Work out the finished part from the listing and answer in its coordinate system (mm). Give positions to 0.01 mm unless a question says otherwise; leave off trailing zeros. Write each loop counter-clockwise with the first axis right and the second up, starting at its lowest first coordinate (ties: lowest second). Pieces come first, ordered by that corner, then holes. Notation, with made-up numbers: (15.5, 60) -> (38.5, 60) arc R19 cw to (38.5, 68) -> close; hole circle Ø3 at (-21.75, 88). An arc over 180 degrees is marked (long way). Use a Markdown table: item, result. Add a question column.
Q1. Section D-D, the plane z = 19.5 is taken. Give the vertices of the cut face in (x, y), plus the area to 3 significant figures.
Q2. Each of these flat-tipped pins is pushed along its axis until it touches: pin 1 Ø5.5 at (x, y) = (17.5, -51) entering from -Z; pin 2 Ø5.5 at (y, z) = (1, -116) entering from -X; pin 3 Ø5.5 at (y, z) = (-50.5, -151.5) entering from +X; pin 4 Ø10 at (x, z) = (-24.5, -42.5) entering from +Y. Where does it stop, or does it pass through?
Q3. Section A-A, the plane y = -44 is taken. Give the vertices of the cut face in (x, z).
Q4. Section C-C, the plane x = 19 is taken. State how many separate pieces and enclosed holes the cut face has, plus the area to 3 significant figures.
Q5. Consider line 1 (Z direction, x = 0, y = 1); line 2 (Z direction, x = 0, y = -35.25); line 3 (X direction, y = -17, z = 0). Determine where each line is inside the solid, lowest interval first.
Q6. Section B-B, the plane z = -150 is taken. Give the vertices of the cut face in (x, y).
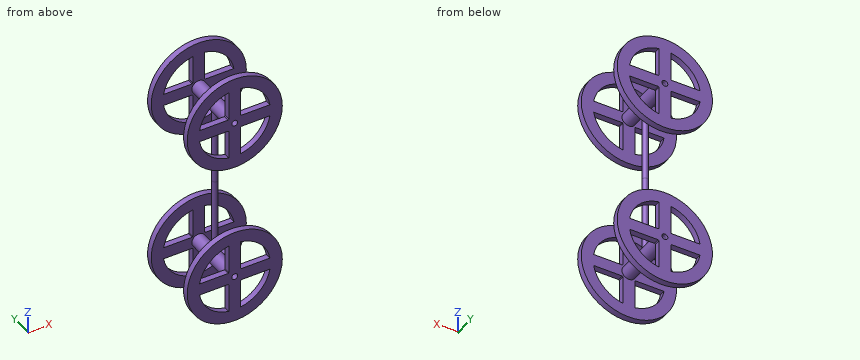
from build123d import *

# Parameters (mm, degrees)
F0_R     = 40
F1_DEPTH = 2.5
F2_R     = 5.8113961387
F2_R_2   = 3.4738590418
F3_DEPTH = 25


with BuildPart() as f1:
    # F0 (on Front) → F1 (new body, symmetric)
    with BuildSketch(Plane.XZ):
        Circle(F0_R)
        with BuildLine():
            Line((-29.5803989155, -5), (-5.5901699437, -5))
            ThreePointArc((-5.5901699437, -5), (-5.3033008589, -5.3033008589), (-5, -5.5901699437))
            Line((-5, -5.5901699437), (-5, -29.5803989155))
            ThreePointArc((-5, -29.5803989155), (-21.2132034356, -21.2132034356), (-29.5803989155, -5))
        make_face(mode=Mode.SUBTRACT)
        with BuildLine():
            Line((5, -29.5803989155), (5, -5.5901699437))
            ThreePointArc((5, -5.5901699437), (5.3033008589, -5.3033008589), (5.5901699437, -5))
            Line((5.5901699437, -5), (29.5803989155, -5))
            ThreePointArc((29.5803989155, -5), (21.2132034356, -21.2132034356), (5, -29.5803989155))
        make_face(mode=Mode.SUBTRACT)
        with BuildLine():
            Line((-5, 29.5803989155), (-5, 5.5901699437))
            ThreePointArc((-5, 5.5901699437), (-5.3033008589, 5.3033008589), (-5.5901699437, 5))
            Line((-5.5901699437, 5), (-29.5803989155, 5))
            ThreePointArc((-29.5803989155, 5), (-21.2132034356, 21.2132034356), (-5, 29.5803989155))
        make_face(mode=Mode.SUBTRACT)
        with BuildLine():
            ThreePointArc((0, -2.5), (-1.767766953, 1.767766953), (2.5, 0))
            ThreePointArc((2.5, 0), (1.767766953, -1.767766953), (0, -2.5))
        make_face(mode=Mode.SUBTRACT)
        with BuildLine():
            ThreePointArc((5, 29.5803989155), (21.2132034356, 21.2132034356), (29.5803989155, 5))
            Line((29.5803989155, 5), (5.5901699437, 5))
            ThreePointArc((5.5901699437, 5), (5.3033008589, 5.3033008589), (5, 5.5901699437))
            Line((5, 5.5901699437), (5, 29.5803989155))
        make_face(mode=Mode.SUBTRACT)
    extrude(amount=F1_DEPTH, both=True)

    # F2 (on Front) → F3 (join)
    with BuildSketch(Plane.XZ):
        Circle(F2_R)
        Circle(F2_R_2, mode=Mode.SUBTRACT)
    extrude(amount=F3_DEPTH)

    # F4: F1 across face


with BuildPart() as f1_1:
    add(f1.part)
    add(f1.part.mirror(Plane.XZ.offset(25)))

    # F6 (on offset) → F7 (revolve)
    with BuildSketch(Plane.XZ.offset(25)):
        with BuildLine():
            Line((0, -2.6413043961), (0, -69.5543512702))
            Line((0, -69.5543512702), (2.3478262592, -69.5543512702))
            Line((2.3478262592, -69.5543512702), (2.3478262592, -2.6413043961))
            Line((2.3478262592, -2.6413043961), (2.3478262592, -1.2100416395))
            ThreePointArc((2.3478262592, -1.2100416395), (1.3748455569, -2.2552801616), (0, -2.6413043961))
        make_face()
    revolve(axis=Axis((0, -25, -36.0978278331), (0, 0, -1)))

    # F8: F1 across face


with BuildPart() as f1_2:
    add(f1_1.part)
    add(f1_1.part.mirror(Plane(origin=(0, -25, -69.5543512702), x_dir=(1, 0, 0), z_dir=(0, 0, -1))))


solid = f1_2.part
Result set:
| question | item | result |
|---|---|---|
| 1 | outline | (-34.92, -52.5) -> (-22.8, -52.5) -> (-22.8, -47.5) -> (-34.92, -47.5) -> close; (-34.92, -2.5) -> (-22.8, -2.5) -> (-22.8, 2.5) -> (-34.92, 2.5) -> close; (-5, -52.5) -> (5, -52.5) -> (5, -47.5) -> (-5, -47.5) -> close; (-5, -2.5) -> (5, -2.5) -> (5, 2.5) -> (-5, 2.5) -> close; (22.8, -52.5) -> (34.92, -52.5) -> (34.92, -47.5) -> (22.8, -47.5) -> close; (22.8, -2.5) -> (34.92, -2.5) -> (34.92, 2.5) -> (22.8, 2.5) -> close |
| 1 | area | 343 mm2 |
| 2 | pin 1 | stops at z = -176.29 |
| 2 | pin 2 | stops at x = -34.43 |
| 2 | pin 3 | stops at x = 38.82 |
| 2 | pin 4 | passes through |
| 3 | outline | circle Ø11.62 at (0, -139.11); circle Ø11.62 at (0, 0); hole circle Ø6.95 at (0, -139.11); hole circle Ø6.95 at (0, 0) |
| 4 | separate pieces | 12 |
| 4 | enclosed holes | 0 |
| 4 | area | 679 mm2 |
| 5 | line 1 | z = -179.11 to -141.61, -136.61 to -99.11, -40 to -2.5, 2.5 to 40 |
| 5 | line 2 | z = -144.92 to -142.58, -135.63 to -133.3, -5.81 to -3.47, 3.47 to 5.81 |
| 5 | line 3 | x = -5.81 to -3.47, 3.47 to 5.81 |
| 6 | outline | (-38.49, -52.5) -> (-27.95, -52.5) -> (-27.95, -47.5) -> (-38.49, -47.5) -> close; (-38.49, -2.5) -> (-27.95, -2.5) -> (-27.95, 2.5) -> (-38.49, 2.5) -> close; (-5, -52.5) -> (5, -52.5) -> (5, -47.5) -> (-5, -47.5) -> close; (-5, -2.5) -> (5, -2.5) -> (5, 2.5) -> (-5, 2.5) -> close; (27.95, -52.5) -> (38.49, -52.5) -> (38.49, -47.5) -> (27.95, -47.5) -> close; (27.95, -2.5) -> (38.49, -2.5) -> (38.49, 2.5) -> (27.95, 2.5) -> close |
